Could you check a few things on this model? Use its own coordinates, in mm. Face numbers are marked on the shaded views. A direction names the side the tool comes from. Coordinates: 2 decimals unless noted, no trailing zeros. Loops run counter-clockwise (first coordinate to the right, second up) from the corner with the lowest first, then second, coordinate; pieces in that order, holes last. Notation, with made-up numbers: (-40, -33.75) - (-6, -33.75) arc R17 cw to (-6, -27.75) - close; hole circle Ø8 at (52.25, -33). An arc over 180 degrees is marked (long way). Put each result on its own line as item: value. Start each with the question number.
```python
from build123d import *

# Parameters (mm, degrees)
SKETCH1_R           = 7.97
MOTOR_DEPTH         = 5
SHAFT_FOR_PROP_R    = 0.75
BOSS_EXTRUDE2_DEPTH = 4.8
SKETCH3_R           = 2.5
BOSS_EXTRUDE3_DEPTH = 2
SKETCH5_R           = 1
BOSS_EXTRUDE4_DEPTH = 2


with BuildPart() as part:
    # Sketch1 → motor (new body)
    with BuildSketch(Plane.XY):
        Circle(SKETCH1_R)
    extrude(amount=MOTOR_DEPTH)

    # shaft for prop → Boss-Extrude2 (add)
    with BuildSketch(Plane.XY.offset(5)):
        Circle(SHAFT_FOR_PROP_R)
    extrude(amount=BOSS_EXTRUDE2_DEPTH)

    # Sketch3 → Boss-Extrude3 (add)
    with BuildSketch(Plane(origin=(0, 0, 0), x_dir=(-1, 0, 0), z_dir=(0, 0, -1))):
        Circle(SKETCH3_R)
    extrude(amount=BOSS_EXTRUDE3_DEPTH)

    # Sketch5 → Boss-Extrude4 (add)
    with BuildSketch(Plane(origin=(0, 0, -2), x_dir=(-1, 0, 0), z_dir=(0, 0, -1))):
        with BuildLine():
            ThreePointArc((-4.5, 2), (-6.5, 0), (-4.5, -2))
            ThreePointArc((-4.5, -2), (-2.732233047, -2.732233047), (-2, -4.5))
            ThreePointArc((-2, -4.5), (0, -6.5), (2, -4.5))
            ThreePointArc((2, -4.5), (2.732233047, -2.732233047), (4.5, -2))
            ThreePointArc((4.5, -2), (6.5, 0), (4.5, 2))
            ThreePointArc((4.5, 2), (2.732233047, 2.732233047), (2, 4.5))
            ThreePointArc((2, 4.5), (0, 6.5), (-2, 4.5))
            ThreePointArc((-2, 4.5), (-2.732233047, 2.732233047), (-4.5, 2))
        make_face()
        with Locations((4.5, 0)):
            Circle(SKETCH5_R, mode=Mode.SUBTRACT)
        with Locations((-4.5, 0)):
            Circle(SKETCH5_R, mode=Mode.SUBTRACT)
        with Locations((0, -4.5)):
            Circle(SKETCH5_R, mode=Mode.SUBTRACT)
        with Locations((0, 4.5)):
            Circle(SKETCH5_R, mode=Mode.SUBTRACT)
    extrude(amount=BOSS_EXTRUDE4_DEPTH)


solid = part.part
```
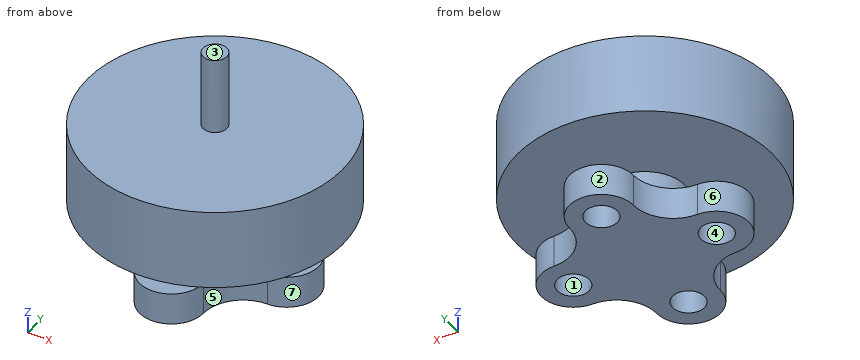
(1) If we mould it in two halves opening along X, with no side actions, what happens to the marked faces 1, 2, 3 and 4? For each: pulls with the +X half, pulls with the -X half, needs draft (parallel to the pull), parting line crosses it, or undercut.
(2) I need wall thicknesses on L1, parallel to Y at x = -4.5, z = -2.9; L2, parallel to Z at x = -1, y = -4.25; L3, parallel to Z at x = 2.5, y = 5.5. Which ranges of each line are inside material? Lowest first, please. Write a range as [from, to].
(3) For pin 1 Ø3 at (y, z) = (6, 4.5) entering from +X; pin 2 Ø1.2 at (x, y) = (0, -4.5) entering from +Z; pin 3 Ø1.2 at (x, y) = (0, 4.5) entering from -Z, each with a flat end and sliding along its axis, tell me the tip position at first contact or that it passes through.
(4) Which directions (+Z, -Z, +X, -X, +Y, -Y) give clear straight access to the entire face, cutting with the end or side of a thin tool? Please do the marked faces 5, 6 and 7.
(5) I want a section at A-A on y = 0. List the corners of the cut face in (x, z) for me.
(6) I want a section at D-D on x = -6.25. List the corners of the cut face in (y, z) for me, and give its area (3 significant figures).
(7) I want a section at C-C on y = 6. List the corners of the cut face in (x, z) for me.
Answer sheet:
1. face 1: undercut
1. face 2: parting line crosses it
1. face 3: needs draft
1. face 4: undercut
2. L1: y = [-2, -1], [1, 2]
2. L2: z = [-4, -2], [0, 5]
2. L3: z = [0, 5]
3. pin 1: stops at x = 6.58
3. pin 2: stops at z = 5
3. pin 3: stops at z = 0
4. face 5: -Z, +X, -Y
4. face 6: -Z, -X
4. face 7: -Z, +X
5. outline: (-7.97, 0) - (-2.5, 0) - (-2.5, -2) - (-3.5, -2) - (-3.5, -4) - (3.5, -4) - (3.5, -2) - (2.5, -2) - (2.5, 0) - (7.97, 0) - (7.97, 5) - (0.75, 5) - (0.75, 9.8) - (-0.75, 9.8) - (-0.75, 5) - (-7.97, 5) - close; (-6.5, -4) - (-5.5, -4) - (-5.5, -2) - (-6.5, -2) - close; (5.5, -4) - (6.5, -4) - (6.5, -2) - (5.5, -2) - close
6. outline: (-4.95, 0) - (4.95, 0) - (4.95, 5) - (-4.95, 5) - close; (-0.97, -4) - (0.97, -4) - (0.97, -2) - (-0.97, -2) - close
6. area: 53.3 mm^2
7. outline: (-5.25, 0) - (5.25, 0) - (5.25, 5) - (-5.25, 5) - close; (-1.32, -4) - (1.32, -4) - (1.32, -2) - (-1.32, -2) - close
